Study the drawing (mm; zero at the part's minimum x, y, z) and answer. A direction names the side the tool comes from. Give positions to 0.01 mm unless a question says otherwise; leave off trailing zeros. Order: outer loops, then holes, each group sorted by start corner. A loop starts at its lowest first (then second) coordinate and runs counter-clockwise, first axis right, second up. Notation, with made-up numbers: (-26, 16.5) -> (8, 16.5) arc R24 cw to (8, 35.5) -> close; hole circle Ø9 at (-20, 17). An arc over 180 degrees is marked (long way). Answer as CSV lines item,"result". Start each with the question number.
1. A cutting plane is placed at C-C (x = 40). Give the vertices of the cut face in (y, z), then the cut area to 4 significant figures.
2. A cutting plane is placed at A-A (z = 5). Give the vertices of the cut face in (x, y), then the cut area to 3 significant figures.
3. Find the intervals of material crossed by L1, parallel to X at y = 6.5, z = 15; L2, parallel to X at y = 13.5, z = 19; L3, parallel to X at y = 25, z = 17.75, in increasing order.
4. For the marked faces 5, 6, 7, 8 and 9, determine the directions among +Z, -Z, +X, -X, +Y, -Y from which every point of the face is accessible in a straight line to the end or side of a thin tool.
5. A cutting plane is placed at B-B (y = 17.5). Give the vertices of the cut face in (x, z).
6. A cutting plane is placed at D-D (x = 74). Give the vertices of the cut face in (y, z), then the cut area to 3 significant figures.
7. For a pull along X with two mould halves and no side action, classify the marked faces 1, 2, 3 and 4 as released by +X, released by -X, zero draft, split by the parting line, or undercut.
8. Flat-ended cylindrical pins translate along their axes: pin 1 (5 mm diameter, centred on x = 56.5, z = 16, fed in from +Y) (1 decimal); pin 2 (4 mm diameter, centred on y = 38.5, z = 6, fed in from -X); pin 3 (7.5 mm diameter, centred on x = 74, z = 10.5, fed in from +Y). Find the tip coordinate at first contact, or state that the pin passes through.
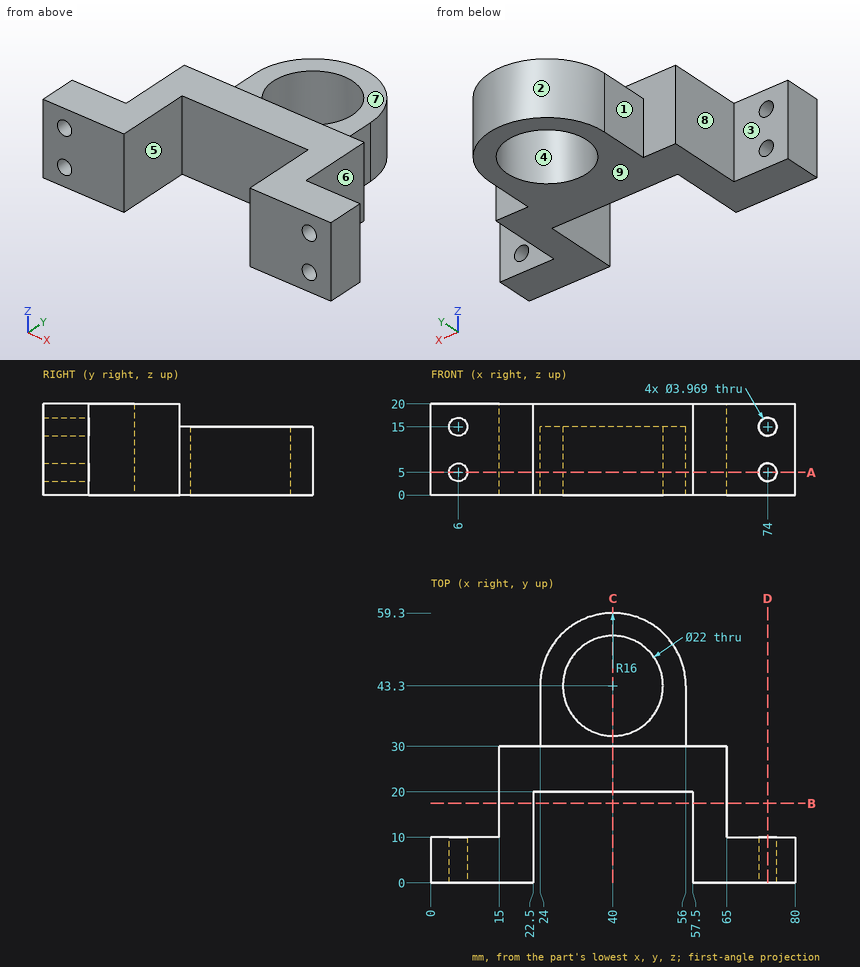
Answer sheet:
1,outline,"(20, 0) -> (32.3, 0) -> (32.3, 15) -> (30, 15) -> (30, 20) -> (20, 20) -> close; (54.3, 0) -> (59.3, 0) -> (59.3, 15) -> (54.3, 15) -> close"
1,area,"309.5 mm^2"
2,outline,"(0, 0) -> (4.02, 0) -> (4.02, 10) -> (0, 10) -> close; (7.98, 0) -> (22.5, 0) -> (22.5, 20) -> (57.5, 20) -> (57.5, 0) -> (72.02, 0) -> (72.02, 10) -> (65, 10) -> (65, 30) -> (56, 30) -> (56, 43.3) arc R16 ccw to (24, 43.3) -> (24, 30) -> (15, 30) -> (15, 10) -> (7.98, 10) -> close; (75.98, 0) -> (80, 0) -> (80, 10) -> (75.98, 10) -> close; hole circle Ø22 at (40, 43.3)"
2,area,"1,470 mm^2"
3,L1,"x = 0 to 4.02, 7.98 to 22.5, 57.5 to 72.02, 75.98 to 80"
3,L2,"x = 15 to 22.5, 57.5 to 65"
3,L3,"x = 15 to 65"
4,face 5,"+Z, -Z, -Y"
4,face 6,"+Z, -Z, +X, +Y"
4,face 7,"+Z, +X, -X, +Y"
4,face 8,"+Z, -Z, -X, +Y"
4,face 9,"-Z, +X, -X, +Y, -Y"
5,outline,"(15, 0) -> (22.5, 0) -> (22.5, 20) -> (15, 20) -> close; (57.5, 0) -> (65, 0) -> (65, 20) -> (57.5, 20) -> close"
6,outline,"(0, 0) -> (10, 0) -> (10, 3.02) -> (0, 3.02) -> close; (0, 6.98) -> (10, 6.98) -> (10, 13.02) -> (0, 13.02) -> close; (0, 16.98) -> (10, 16.98) -> (10, 20) -> (0, 20) -> close"
6,area,"121 mm^2"
7,face 1,"released by -X"
7,face 2,"split by the parting line"
7,face 3,"zero draft"
7,face 4,"undercut"
8,pin 1,"stops at y = 50.7"
8,pin 2,"stops at x = 24"
8,pin 3,"stops at y = 10"
